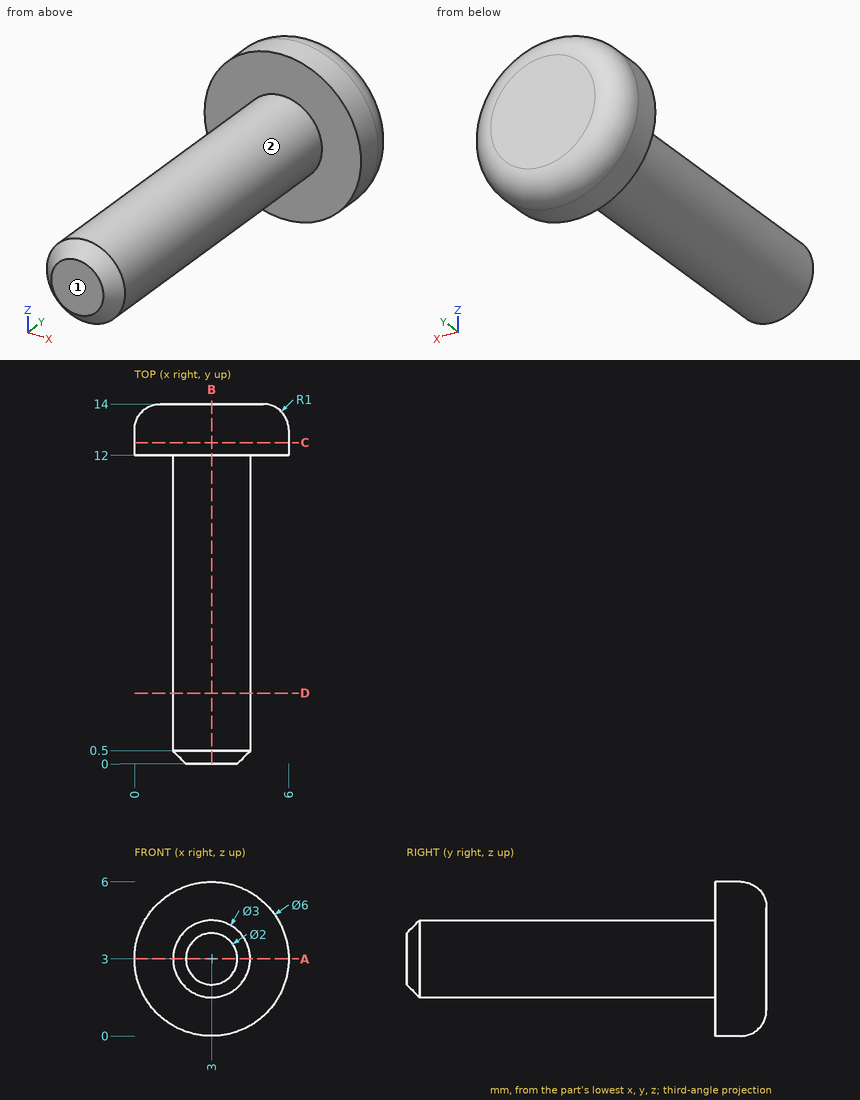
Input: dimensioned drawing with shaded views. Units: mm. Origin: part minimum x, y, z. A direction names the side the tool comes from. Round coordinates to 2 decimals unless told otherwise and drop trailing zeros. Loops run counter-clockwise (first coordinate to the right, second up) from the corner with the lowest first, then second, coordinate; pieces in that order, holes last.
1) Pin query (flat end, axial travel): pin 1 (1 mm diameter, centred on y = 4, z = 4.5, fed in from +X); pin 2 (3 mm diameter, centred on y = 3.5, z = 4, fed in from -X). Return the tip coordinate at first contact, or that it passes through.
Ans:
pin 1: stops at x = 4.12
pin 2: stops at x = 1.5
2) Section query D-D on y = 2.75. Return the cut outline in (x, z).
Ans:
outline: circle Ø3 at (3, 3)
3) Section query A-A on z = 3. Return the cut outline in (x, y).
Ans:
outline: (0, 12) - (1.5, 12) - (1.5, 0.5) - (2, 0) - (4, 0) - (4.5, 0.5) - (4.5, 12) - (6, 12) - (6, 13) arc R1 ccw to (5, 14) - (1, 14) arc R1 ccw to (0, 13) - close
4) Set-up query: the marked faces 1 and 2. Return all of +Z, -Z, +X, -X, +Y, -Y with unobstructed straight access to the full face (end or side cutting, diameter ignored); none if empty.
Ans:
face 1: +Z, -Z, +X, -X, -Y
face 2: -Y
5) Section query B-B on x = 3. Return the cut outline in (y, z).
Ans:
outline: (0, 2) - (0.5, 1.5) - (12, 1.5) - (12, 0) - (13, 0) arc R1 ccw to (14, 1) - (14, 5) arc R1 ccw to (13, 6) - (12, 6) - (12, 4.5) - (0.5, 4.5) - (0, 4) - close
6) Material intervals for line 1 (Y direction, x = 3.7, z = 1.5); line 2 (X direction, y = 5, z = 4); line 3 (Z direction, x = 0.3, y = 13), sorted ascending.
Ans:
line 1: y = 12 to 14
line 2: x = 1.88 to 4.12
line 3: z = 1.69 to 4.31
7) Section query C-C on y = 12.5. Return the cut outline in (x, z), plus the area to 3 significant figures.
Ans:
outline: circle Ø6 at (3, 3)
area: 28.3 mm2
